Autodesk Inventor part; units mm, degrees
ref_plane "YZ Plane" through (0, 0, 0) normal (1, 0, 0) x (0, 1, 0)
ref_plane "XZ Plane" through (0, 0, 0) normal (0, 1, 0) x (-1, 0, 0)
ref_plane "XY Plane" through (0, 0, 0) normal (0, 0, 1) x (1, 0, 0)
sketch "草图22" plane through (0, 0, 0) normal (0, 0, 1) x (1, 0, 0)
  line L0 (32.055, -44.6465) -> (-32.055, -44.6465)
  line L1 (-32.055, -44.6465) -> (-32.055, 44.6465)
  line L2 (-32.055, 44.6465) -> (32.055, 44.6465)
  line L3 (32.055, 44.6465) -> (32.055, -44.6465)
  line L4 (32.055, -44.6465) -> (-32.055, 44.6465) construction
  line L5 (-32.055, -44.6465) -> (32.055, 44.6465) construction
  line L6 (24.394, -19.5595) -> (-24.107, -19.5595) construction
  line L7 (-24.107, -19.5595) -> (-24.107, 4.4405) construction
  line L8 (-24.107, 4.4405) -> (24.394, 4.4405) construction
  line L9 (24.394, 4.4405) -> (24.394, -19.5595) construction
  line L10 (24.394, -19.5595) -> (-24.107, 4.4405) construction
  line L11 (-24.107, -19.5595) -> (24.394, 4.4405) construction
  circle A0 centre (-24.107, 4.4405) radius 1.7
  circle A1 centre (-24.107, -19.5595) radius 1.7
  circle A2 centre (24.394, -19.5595) radius 1.7
  circle A3 centre (24.394, 4.4405) radius 1.7
  point P0 (0, 0)
  point P1 (-14.525, 44.6465)
  point P2 (3.476, 44.6465)
  point P3 (0.1435, -7.5595)
  dimension "d101" = 89.293
  dimension "d102" = 64.11
  dimension "d103" = 7.661
  dimension "d104" = 7.948
  dimension "d105" = 25.087
  dimension "d106" = 40.206
  dimension "d107" = 17.53
  dimension "d108" = 28.579
  dimension "d109" = 3.4
  dimension "d110" = 3.4
  dimension "d111" = 3.4
  dimension "d112" = 3.4
extrude "拉伸18" add sketch "草图22" along normal blind 1
sketch "草图23" plane through (0, 0, 1) normal (0, 0, 1) x (1, 0, 0)
  circle A0 centre (-24.107, 4.4405) radius 1.7
  circle A1 centre (24.394, 4.4405) radius 1.7
  circle A2 centre (24.394, -19.5595) radius 1.7
  circle A3 centre (-24.107, -19.5595) radius 1.7
  line L0 (32.055, 44.6465) -> (-32.055, 44.6465)
  line L1 (-32.055, -44.6465) -> (32.055, -44.6465)
  line L2 (-32.055, 44.6465) -> (32.055, 44.6465)
  line L3 (32.055, 44.6465) -> (32.055, -44.6465)
  line L4 (32.055, -44.6465) -> (-32.055, -44.6465)
  line L5 (-32.055, -44.6465) -> (-32.055, 44.6465)
  circle A4 centre (24.394, 4.4405) radius 3.05
  circle A5 centre (24.394, -19.5595) radius 1.7
  circle A6 centre (24.394, -19.5595) radius 3.05
  circle A7 centre (-24.107, -19.5595) radius 3.05
  circle A8 centre (-24.107, 4.4405) radius 3.05
  point P0 (0, 0)
  dimension "d164" = 6.1
extrude "拉伸19" add sketch "草图23" along normal blind 2 contours L3 L1 L5 L0
sketch "草图25" plane through (0, 0, 3) normal (0, 0, 1) x (1, 0, 0)
  circle A0 centre (-23.869, 38.3445) radius 2.7
  circle A1 centre (-23.869, 31.3595) radius 2.7
  circle A2 centre (-23.869, 24.5015) radius 2.7
  line L0 (32.055, 44.6465) -> (-32.055, 44.6465)
  line L1 (-32.055, 44.6465) -> (-32.055, -44.6465)
  circle A3 centre (12.608, 39.1095) radius 2.5
  line L2 (32.055, -44.6465) -> (32.055, 44.6465)
  circle A4 centre (12.608, 30.2185) radius 2.5
  circle A5 centre (12.608, 21.3885) radius 2.5
  circle A6 centre (21.582, 21.3885) radius 2.5
  circle A7 centre (28.639, 26.6255) radius 1
  circle A8 centre (28.639, 23.2155) radius 1
  line L3 (7.225, 20.5575) -> (-18.275, 20.5575) construction
  line L4 (-18.275, 20.5575) -> (-18.275, 47.0575) construction
  line L5 (-18.275, 47.0575) -> (7.225, 47.0575) construction
  line L6 (7.225, 47.0575) -> (7.225, 20.5575) construction
  line L7 (-18.775, 25.0575) -> (7.725, 25.0575)
  line L8 (7.725, 25.0575) -> (7.725, 43.0575)
  line L9 (-18.775, 43.0575) -> (-18.775, 25.0575)
  line L10 (-10.025, 43.0575) -> (-10.025, 47.0575)
  line L11 (-10.025, 47.0575) -> (-5.525, 47.0575)
  line L12 (-1.025, 43.0575) -> (-1.025, 47.0575)
  line L13 (-1.025, 47.0575) -> (-5.525, 47.0575)
  line L14 (7.725, 43.0575) -> (-1.025, 43.0575)
  line L15 (-10.025, 43.0575) -> (-18.775, 43.0575)
  point P0 (0, 0)
  point P1 (-5.525, 21.0575)
  point P2 (-5.525, 20.5575)
  dimension "d123" = 5.4
  dimension "d124" = 5.4
  dimension "d125" = 5.4
  dimension "d126" = 6.302
  dimension "d127" = 8.186
  dimension "d128" = 8.186
  dimension "d129" = 8.186
  dimension "d130" = 13.287
  dimension "d131" = 20.145
  dimension "d132" = 5.537
  dimension "d133" = 19.447
  dimension "d134" = 5
  dimension "d135" = 5
  dimension "d136" = 14.428
  dimension "d137" = 19.447
  dimension "d138" = 5
  dimension "d139" = 19.447
  dimension "d140" = 23.258
  dimension "d141" = 5
  dimension "d142" = 23.258
  dimension "d143" = 10.473
  dimension "d144" = 2
  dimension "d145" = 2
  dimension "d146" = 3.416
  dimension "d147" = 3.416
  dimension "d148" = 18.021
  dimension "d149" = 3.41
  dimension "d150" = 26.53
  dimension "d151" = 23.589
  dimension "d152" = 0.5
  dimension "d153" = 26.53
  dimension "d154" = 26.5
  dimension "d155" = 25.5
  dimension "d156" = 4.5
  dimension "d158" = 0.5
  dimension "d159" = 0.5
extrude "拉伸21" cut sketch "草图25" against normal up to next
sketch "草图26" plane through (0, 0, 3) normal (0, 0, 1) x (1, 0, 0)
  circle A0 centre (-24.107, 4.4405) radius 1.7
  circle A1 centre (-24.107, -19.5595) radius 1.7
  circle A2 centre (24.394, 4.4405) radius 1.7
  circle A3 centre (24.394, -19.5595) radius 1.7
  line L0 (1.394, -6.2595) -> (11.894, -6.2595)
  line L1 (11.894, -6.2595) -> (11.894, -21.2595)
  line L2 (11.894, -21.2595) -> (1.394, -21.2595)
  line L3 (1.394, -21.2595) -> (1.394, -6.2595)
  line L4 (-24.107, -19.5595) -> (24.394, -19.5595) construction
  line L5 (32.055, -44.6465) -> (32.055, 44.6465) construction
  line L6 (24.394, -21.2595) -> (-24.107, -21.2595) construction
  point P0 (0, 0)
  dimension "d165" = 12.5
  dimension "d166" = 23
  dimension "d167" = 15
extrude "拉伸22" cut sketch "草图26" against normal through all contours L0 L1 L2 L3
sketch "草图27" plane through (0, 0, 0) normal (0, 0, -1) x (-1, 0, 0)
  line L0 (10.855, 21.0575) -> (0.195, 21.0575)
  line L1 (0.195, 21.0575) -> (0.195, 23.5575)
  line L2 (0.195, 23.5575) -> (10.855, 23.5575)
  line L3 (10.855, 23.5575) -> (10.855, 21.0575)
  line L4 (10.025, 44.6465) -> (32.055, 44.6465)
  line L5 (32.055, 44.6465) -> (32.055, -44.6465)
  point P0 (0, 0)
  dimension "d170" = 23.589
  dimension "d171" = 21.089
  dimension "d172" = 21.2
  dimension "d173" = 31.86
extrude "拉伸23" cut sketch "草图27" against normal blind 2.8
sketch "草图28" plane through (0, 0, 3) normal (0, 0, 1) x (1, 0, 0)
  line L0 (-32.055, -44.6465) -> (32.055, -44.6465)
  line L1 (-29.408, -44.6465) -> (29.212, -44.6465)
  line L2 (29.212, -44.6465) -> (29.212, -34.7635)
  line L3 (29.212, -34.7635) -> (-29.408, -34.7635)
  line L4 (-29.408, -34.7635) -> (-29.408, -44.6465)
  line L5 (32.055, -44.6465) -> (32.055, 44.6465)
  line L6 (-32.055, 44.6465) -> (-32.055, -44.6465)
  point P0 (0, 0)
  point P1 (29.212, -44.6465)
  dimension "d176" = 2.843
  dimension "d177" = 2.647
  dimension "d178" = 9.883
extrude "拉伸24" cut sketch "草图28" against normal through all
sketch "草图29" plane through (0, 0, 0) normal (0, 0, -1) x (-1, 0, 0)
  line L0 (29.408, -34.7635) -> (-29.212, -34.7635)
  line L1 (29.408, -34.7635) -> (-29.212, -34.7635)
  line L2 (-29.212, -34.7635) -> (-29.212, -32.7635)
  line L3 (-29.212, -32.7635) -> (29.408, -32.7635)
  line L4 (29.408, -32.7635) -> (29.408, -34.7635)
  point P0 (0, 0)
  point P1 (-29.212, -34.7635)
  dimension "d181" = 2
extrude "拉伸25" add sketch "草图29" along normal blind 3
sketch "草图30" plane through (0, 0, 0) normal (0, 0, -1) x (-1, 0, 0)
  line L0 (29.408, -32.7635) -> (29.408, -34.7635)
  line L1 (32.055, 44.6465) -> (32.055, -44.6465)
  line L2 (29.408, -32.7635) -> (32.055, -32.7635)
  line L3 (32.055, -32.7635) -> (32.055, -44.6465)
  line L4 (32.055, -44.6465) -> (29.408, -44.6465)
  line L5 (29.408, -44.6465) -> (29.408, -32.7635)
  line L6 (-29.212, -34.7635) -> (-29.212, -32.7635)
  line L7 (-32.055, -44.6465) -> (-32.055, 44.6465)
  line L8 (-29.212, -32.7635) -> (-32.055, -32.7635)
  line L9 (-32.055, -32.7635) -> (-32.055, -44.6465)
  line L10 (-32.055, -44.6465) -> (-29.212, -44.6465)
  line L11 (-29.212, -44.6465) -> (-29.212, -32.7635)
  point P0 (0, 0)
extrude "拉伸26" add sketch "草图30" along normal blind 11.5
sketch "草图31" plane through (0, 0, 0) normal (0, 0, -1) x (-1, 0, 0)
  line L0 (-32.055, -32.7635) -> (-32.055, 44.6465)
  line L1 (32.055, 44.6465) -> (32.055, -32.7635)
  line L2 (-33.555, 44.6465) -> (-33.555, -44.6465)
  line L3 (-32.055, -44.6465) -> (-32.055, 44.6465)
  line L4 (33.555, 44.6465) -> (33.555, -44.6465)
  line L5 (32.055, -44.6465) -> (32.055, 44.6465)
  line L6 (-32.055, 44.6465) -> (32.055, 44.6465)
  line L7 (33.555, 44.6465) -> (33.555, 46.1465)
  line L8 (33.555, 46.1465) -> (-33.555, 46.1465)
  line L9 (-33.555, 46.1465) -> (-33.555, 44.6465)
  line L10 (29.408, -44.6465) -> (32.055, -44.6465)
  line L11 (33.555, -44.6465) -> (33.555, -46.1465)
  line L12 (33.555, -46.1465) -> (29.408, -46.1465)
  line L13 (29.408, -46.1465) -> (29.408, -44.6465)
  line L14 (-32.055, -44.6465) -> (-29.212, -44.6465)
  line L15 (-29.212, -44.6465) -> (-29.212, -46.1465)
  line L16 (-29.212, -46.1465) -> (-33.555, -46.1465)
  line L17 (-33.555, -46.1465) -> (-33.555, -44.6465)
  point P0 (0, 0)
  point P1 (-32.055, 44.6465)
  point P2 (32.055, -32.7635)
  dimension "d188" = 1.5
  dimension "d202" = 1.5
extrude "拉伸27" add sketch "草图31" along normal blind 11.5 and the other way blind 3
sketch "草图32" plane through (-33.555, 46.1465, -11.5) normal (0, 1, 0) x (1, 0, 0)
  line L0 (14.78, -11.5) -> (41.28, -11.5)
  line L1 (41.28, -11.5) -> (14.78, -11.5)
  line L2 (14.78, -11.5) -> (14.78, -10.2)
  line L3 (14.78, -10.2) -> (41.28, -10.2)
  line L4 (41.28, -10.2) -> (41.28, -11.5)
  point P0 (33.555, -11.5)
  dimension "d193" = 1.3
extrude "拉伸28" cut sketch "草图32" against normal blind 11
sketch "草图33" plane through (-33.555, 46.1465, -11.5) normal (0, 1, 0) x (1, 0, 0)
  line L0 (65.61, 0) -> (1.5, 0)
  line L1 (17.53, 0) -> (38.5, 0)
  line L2 (38.5, 0) -> (38.5, -1)
  line L3 (38.5, -1) -> (17.53, -1)
  line L4 (17.53, -1) -> (17.53, 0)
  point P0 (33.555, -11.5)
  dimension "d196" = 16.03
  dimension "d197" = 37
  dimension "d198" = 1
extrude "拉伸29" cut sketch "草图33" against normal blind 11
sketch "草图34" plane through (0, 0, 0) normal (0, 0, -1) x (-1, 0, 0)
  line L0 (18.775, 44.6465) -> (32.055, 44.6465)
  line L1 (18.775, 21.0575) -> (18.775, 44.6465)
  line L2 (-7.725, 44.6465) -> (-7.725, 21.0575)
  line L3 (10.855, 21.0575) -> (0.195, 21.0575)
  line L4 (18.775, 20.5575) -> (-7.725, 20.5575)
  line L5 (-7.725, 46.1465) -> (18.775, 46.1465)
  line L6 (-7.725, 44.6465) -> (-7.725, 46.1465)
  line L7 (-7.725, 46.1465) -> (-7.725, 44.6465)
  line L8 (-7.725, 21.0575) -> (-7.725, 20.5575)
  line L9 (18.775, 21.0575) -> (18.775, 20.5575)
  line L10 (18.775, 44.6465) -> (18.775, 46.1465)
  line L11 (-4.945, 46.1465) -> (16.025, 46.1465)
  point P0 (0, 0)
extrude "拉伸30" cut sketch "草图34" against normal blind 1.3
sketch "草图35" plane through (33.555, -46.1465, -11.5) normal (1, 0, 0) x (0, 0, -1)
  line L0 (0, 90.793) -> (0, 13.383)
  line L1 (0, 86.614) -> (-3, 86.614)
  line L2 (-3, 86.614) -> (-3, 76.174)
  line L3 (-3, 76.174) -> (0, 76.174)
  line L4 (0, 76.174) -> (0, 86.614)
  line L5 (-11.5, 90.793) -> (0, 90.793)
  point P0 (-11.5, 46.1465)
  point P1 (-1.5, 86.614)
  point P2 (0, 76.174)
  point P3 (-0.0335, 85.614)
  dimension "d206" = 4.179
  dimension "d207" = 14.619
  dimension "d208" = 3
extrude "拉伸31" cut sketch "草图35" against normal up to surface (1.5 mm away)
sketch "草图37" plane through (0, 0, 0) normal (0, 0, -1) x (-1, 0, 0)
  circle A0 centre (24.107, 4.4405) radius 1.7
  circle A1 centre (24.107, 4.4405) radius 3
  circle A2 centre (24.107, -19.5595) radius 1.7
  circle A3 centre (24.107, -19.5595) radius 3
  circle A4 centre (-24.394, 4.4405) radius 1.7
  circle A5 centre (-24.394, 4.4405) radius 3
  circle A6 centre (-24.394, -19.5595) radius 1.7
  circle A7 centre (-24.394, -19.5595) radius 3
  point P0 (0, 0)
  dimension "d213" = 6
  dimension "d214" = 6
  dimension "d215" = 6
  dimension "d216" = 6
extrude "拉伸33" add sketch "草图37" along normal blind 0.5
sketch "草图38" plane through (0, 0, -11.5) normal (0, 0, -1) x (-1, 0, 0)
  line L0 (-33.555, 30.0275) -> (-33.555, -46.1465)
  line L1 (-33.555, -46.1465) -> (-29.212, -46.1465)
  line L2 (-29.212, -46.1465) -> (-29.212, -32.7635)
  line L3 (-29.212, -32.7635) -> (-32.055, -32.7635)
  line L4 (-32.055, -32.7635) -> (-32.055, 30.0275)
  line L5 (-32.055, 30.0275) -> (-33.555, 30.0275)
  line L6 (-33.555, 40.4675) -> (-32.055, 40.4675)
  line L7 (-32.055, 40.4675) -> (-32.055, 44.6465)
  line L8 (-33.555, 46.1465) -> (-33.555, 40.4675)
  line L9 (-33.555, 40.4675) -> (-32.055, 40.4675)
  line L10 (-32.055, 40.4675) -> (-32.055, 44.6465)
  line L11 (-32.055, 44.6465) -> (-4.945, 44.6465)
  line L12 (-4.945, 44.6465) -> (-4.945, 46.1465)
  line L13 (-4.945, 46.1465) -> (-33.555, 46.1465)
  line L14 (-33.555, 46.1465) -> (-33.555, 40.4675)
  line L15 (16.025, 46.1465) -> (16.025, 44.6465)
  line L16 (16.025, 44.6465) -> (32.055, 44.6465)
  line L17 (32.055, 44.6465) -> (32.055, -32.7635)
  line L18 (32.055, -32.7635) -> (29.408, -32.7635)
  line L19 (29.408, -32.7635) -> (29.408, -46.1465)
  line L20 (29.408, -46.1465) -> (33.555, -46.1465)
  line L21 (33.555, -46.1465) -> (33.555, 46.1465)
  line L22 (33.555, 46.1465) -> (16.025, 46.1465)
  point P0 (0, 0)
extrude "拉伸34" add sketch "草图38" along normal blind 1
properties part number "TES_Controller_V1_Case_Top"
Work out the finished part from the listing and answer in its coordinate system (mm). A direction names the side the tool comes from. Give positions to 0.01 mm unless a question says otherwise; leave off trailing zeros. Order: outer loops, then holes, each group sorted by start corner. A loop starts at its lowest first (then second) coordinate and runs counter-clockwise, first axis right, second up.
1. Section D-D, the plane x = -4 is taken. Determine the outline of the cut face in (y, z).
Result sheet:
outline: (-34.76, -3) - (-32.76, -3) - (-32.76, 0) - (20.56, 0) - (20.56, 1.3) - (21.06, 1.3) - (21.06, 2.8) - (23.56, 2.8) - (23.56, 1.3) - (25.06, 1.3) - (25.06, 3) - (-34.76, 3) - close; (44.65, -10.5) - (46.15, -10.5) - (46.15, -1.3) - (44.65, -1.3) - close; (44.65, 1.3) - (46.15, 1.3) - (46.15, 3) - (44.65, 3) - close
2. Section C-C, the plane z = -4.75 is taken. Determine the outline of the cut face in (x, y) (1 decimal).
Result sheet:
outline: (-33.6, -46.1) - (-29.4, -46.1) - (-29.4, -32.8) - (-32.1, -32.8) - (-32.1, 44.6) - (32.1, 44.6) - (32.1, -32.8) - (29.2, -32.8) - (29.2, -46.1) - (33.6, -46.1) - (33.6, 46.1) - (-33.6, 46.1) - close
3. Section A-A, the plane x = 3 is taken. Determine the outline of the cut face in (y, z).
Result sheet:
outline: (-34.76, -3) - (-32.76, -3) - (-32.76, 0) - (-21.26, 0) - (-21.26, 3) - (-34.76, 3) - close; (-6.26, 0) - (20.56, 0) - (20.56, 1.3) - (25.06, 1.3) - (25.06, 3) - (-6.26, 3) - close; (43.06, 1.3) - (46.15, 1.3) - (46.15, 3) - (43.06, 3) - close; (44.65, -10.5) - (46.15, -10.5) - (46.15, -1.3) - (44.65, -1.3) - close
4. The mould has two halves that part along Y. Classify faces 5 (the cylindrical face through (26.605, -21.587, -0.246)), 6 (the flat face through (-33.555, -1, -5)), 7 (the cylindrical face through (-22.62, 35.95, 1.52)): released by +Y, released by -Y, zero draft, split by the parting line, or undercut.
Result sheet:
face 5: undercut
face 6: zero draft
face 7: undercut
5. For faces 1 (the flat face through (0, -34, -3)), 2 (the cylindrical face through (-22.42, 33.64, 1.52)), 3 (the flat face through (-22.8, -20.9, 1)), 4 (the flat face through (0, 44.646, -6)), determine the directions among +Z, -Z, +X, -X, +Y, -Y from which every point of the face is accessible in a straight line to the end or side of a thin tool.
Result sheet:
face 1: -Z, -Y
face 2: +Z, -Z
face 3: +Z
face 4: -Z
6. Section B-B, the plane y = -8 is taken. Determine the outline of the cut face in (x, z) (3 decimals).
Result sheet:
outline: (-33.555, -12.5) - (-32.055, -12.5) - (-32.055, 0) - (1.394, 0) - (1.394, 3) - (-33.555, 3) - close; (11.894, 0) - (32.055, 0) - (32.055, -12.5) - (33.555, -12.5) - (33.555, 3) - (11.894, 3) - close
7. Each of these flat-tipped pins is pushed along its axis until it touches: P1, Ø4, axis at x = -0.5, z = -7.5, coming from the -Y side; P2, Ø5.5, axis at x = -24.11, y = 4.44, coming from the +Z side; P3, Ø5.5, axis at x = 24.39, y = -19.56, coming from the -Z side; P4, Ø3, axis at x = 24.39, y = 4.44, coming from the +Z side. Where does it stop, or does it pass through?
Result sheet:
P1: stops at y = 44.65
P2: stops at z = 1
P3: stops at z = -0.5
P4: passes through
8. Straight lines are drawn through the part: L1, parallel to Y at x = -2.5, z = 1.5; L2, parallel to Y at x = -24, z = 1.25; L3, parallel to X at y = -30, z = -4 (3 decimals). For each, find the intervals that lie inside material, in ascending order.
Result sheet:
L1: y = -34.76 to 21.06, 23.56 to 25.06, 44.65 to 46.15
L2: y = -34.76 to -22.61, -16.51 to 1.39, 7.49 to 21.8, 27.2 to 28.66, 34.06 to 35.65, 41.04 to 46.15
L3: x = -33.555 to -32.055, 32.055 to 33.555
